Part model, mm, in its own coordinate system. A direction names the side the tool comes from. Round coordinates to 2 decimals unless told otherwise and drop trailing zeros. Loops run counter-clockwise (first coordinate to the right, second up) from the corner with the lowest first, then second, coordinate; pieces in that order, holes last. Notation, with made-up numbers: (-32, 36) - (-25, 36) arc R24 cw to (-25, 49) - close; hole circle Ø3 at (52.25, 4). An arc over 180 degrees is marked (long way). Put each result on its own line as item: value.
from build123d import *

# Parameters (mm, degrees)
SKETCH1_R           = 14.2875
BOSS_EXTRUDE1_DEPTH = 3.175
FILLET1_R           = 12.7
FILLET2_R           = 25.4
FILLET3_R           = 12.7
FILLET4_R           = 12.7


with BuildPart() as part:
    # Sketch1 → Boss-Extrude1 (new body)
    with BuildSketch(Plane.XY):
        with BuildLine():
            ThreePointArc((-5.519049503, -21.528834562), (13.625155959, -17.558637479), (22.225, 0))
            Line((22.225, 0), (22.225, 101.6))
            Line((22.225, 101.6), (4.879081578, 120.154759877))
            Line((4.879081578, 120.154759877), (-223.720918422, 120.154759877))
            Line((-223.720918422, 120.154759877), (-311.078676661, 77.714630478))
            Line((-311.078676661, 77.714630478), (-315.107157175, 75.757514845))
            ThreePointArc((-315.107157175, 75.757514845), (-324.150818676, 48.808615563), (-299.298978098, 35.009448714))
            Line((-299.298978098, 35.009448714), (-199.469861892, 53.896151905))
            Line((-199.469861892, 53.896151905), (-5.519049503, -21.528834562))
        make_face()
        Circle(SKETCH1_R, mode=Mode.SUBTRACT)
        with Locations((-303.430444421, 56.847067884)):
            Circle(SKETCH1_R, mode=Mode.SUBTRACT)
    extrude(amount=BOSS_EXTRUDE1_DEPTH)

    # Fillet1
    fillet1_edges = [part.edges().sort_by_distance(p)[0] for p in [
        (-199.469861892, 53.896151905, 1.5875),
    ]]
    fillet(fillet1_edges, radius=FILLET1_R)

    # Fillet2
    fillet2_edges = [part.edges().sort_by_distance(p)[0] for p in [
        (-223.720918422, 120.154759877, 1.5875),
    ]]
    fillet(fillet2_edges, radius=FILLET2_R)

    # Fillet3
    fillet3_edges = [part.edges().sort_by_distance(p)[0] for p in [
        (22.225, 101.6, 1.5875),
    ]]
    fillet(fillet3_edges, radius=FILLET3_R)

    # Fillet4
    fillet4_edges = [part.edges().sort_by_distance(p)[0] for p in [
        (4.879081578, 120.154759877, 1.5875),
    ]]
    fillet(fillet4_edges, radius=FILLET4_R)


solid = part.part
1. Pin check, flat tips, straight feed: P1, Ø1, axis at y = -4.5, z = 1, coming from the +X side; P2, Ø8, axis at x = -63.5, y = -5, coming from the +Z side; P3, Ø1, axis at x = -22.5, z = 1.5, coming from the -Y side. Stop position of each tip, or through.
A:
P1: stops at x = 21.86
P2: passes through
P3: stops at y = -15.12
2. Band-saw the part on B-B (x = -65). List the corners of the cut face in (y, z) (3 decimals).
A:
outline: (1.603, 0) - (120.155, 0) - (120.155, 3.175) - (1.603, 3.175) - close
3. Tool access for faces 1 (the flat face through (-115, 66, 0)), 2 (the flat face through (-102.13, 16.04, 1.57)): list every direction of +Z, -Z, +X, -X, +Y, -Y with a clear straight run to the whole face (end or side of a thin tool).
A:
face 1: -Z, +X, -X, +Y, -Y
face 2: +Z, -Z, -Y
4. Band-saw the part on C-C (y = 93). List the corners of the cut face in (x, z) (3 decimals), plus the area to 3 significant figures.
A:
outline: (-279.616, 0) - (22.225, 0) - (22.225, 3.175) - (-279.616, 3.175) - close
area: 958 mm²
5. Band-saw the part on A-A (z = 0.8). Give the number of separate pieces and of enclosed holes in the cut face, plus the area to 3 significant figures.
A:
separate pieces: 1
enclosed holes: 2
area: 29,700 mm²
6. Probe line 1 along X through (y, z) = (59.5, 0.6) (3 decimals); line 2 along Y through (x, z) = (-304, 2.95); line 3 along Y through (x, z) = (-201.5, 0.7). List the from-to ranges inside material, lowest first. Write a range as [from, to].
A:
line 1: x = [-325.497, -317.469], [-289.391, 22.225]
line 2: y = [34.63, 42.57], [71.12, 81.15]
line 3: y = [53.42, 120.15]
7. Two-plate mould, pull along X, no slides. Class faces 3 (the flat face through (-115, 66, 3.175)), 4 (the cylindrical face through (13.4, -17.73, 1.57)), 5 (the cylindrical face through (-14.274, 0.628, 1.565)), 6 (the flat face through (13.79, 110.62, 1.57)): pulls with the +X half, pulls with the -X half, needs draft (parallel to the pull), parting line crosses it, or undercut.
A:
face 3: needs draft
face 4: parting line crosses it
face 5: undercut
face 6: pulls with the +X half
